Source: CAD feature listing. Evaluate the final solid. Frame: model axes, mm. Face numbers are marked on the shaded views. A direction names the side the tool comes from. Round coordinates to 2 decimals unless told otherwise and drop trailing zeros. Order: outer loops, then holes, each group sorted by start corner. A loop starts at its lowest first (then second) coordinate and runs counter-clockwise, first axis right, second up. Notation, with made-up numbers: (-35.5, -11) -> (21.5, -11) arc R4 cw to (21.5, -6) -> close; hole circle Ø1 at (80.5, -39.75). An arc over 180 degrees is marked (long way). Answer as CSV lines item,"result".
from build123d import *

# Parameters (mm, degrees)
FILLET1_R     = 10
CHAMFER1_SIZE = 2


with BuildPart() as part:
    # Sketch1 → Revolve1 (revolve)
    with BuildSketch(Plane.XY, mode=Mode.PRIVATE) as revolve1_sk:
        with BuildLine():
            Line((0, 0), (71.656242166, 0))
            ThreePointArc((71.656242166, 0), (75.656242166, 4), (79.656242166, 0))
            Line((79.656242166, 0), (148.568475549, 0))
            Line((148.568475549, 0), (148.568475549, 17))
            Line((148.568475549, 17), (79.656242166, 17))
            ThreePointArc((79.656242166, 17), (75.656242166, 13), (71.656242166, 17))
            Line((71.656242166, 17), (29.293635646, 17))
            ThreePointArc((29.293635646, 17), (20.349363736, 15.987177379), (11.858039872, 13))
            Line((11.858039872, 13), (-31.431524451, 13))
            Line((-31.431524451, 13), (-31.431524451, 0))
            Line((-31.431524451, 0), (0, 0))
        make_face()
    revolve(revolve1_sk.sketch.rotate(Axis((0, 0, 0), (1, 0, 0)), 90), axis=Axis((0, 0, 0), (1, 0, 0)))

    # Fillet1
    fillet1_edges = [part.edges().sort_by_distance(p)[0] for p in [
        (11.858039872, 0, -13),
        (-31.431524451, 0, -13),
    ]]
    fillet(fillet1_edges, radius=FILLET1_R)

    # Chamfer1
    chamfer1_edges = [part.edges().sort_by_distance(p)[0] for p in [
        (148.568475549, 0, -17),
    ]]
    chamfer(chamfer1_edges, length=CHAMFER1_SIZE)


solid = part.part
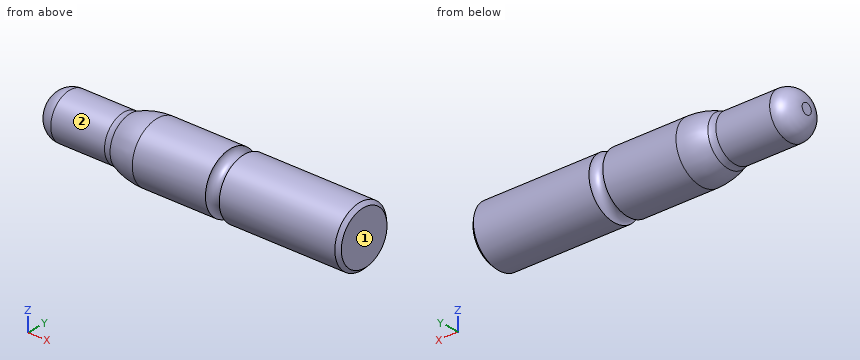
1. Reachability of the marked faces 1 and 2 from +Z, -Z, +X, -X, +Y, -Y: full face, straight path, thin tool, end or side. Return the list, or none.
Results below:
face 1,"+Z, -Z, +X, +Y, -Y"
face 2,"-X"
2. Section query A-A on x = 43. Return loops of the section in (y, z).
Results below:
outline,"circle Ø34 at (0, 0)"
3. Pin query (flat end, axial travel): pin 1 (6 mm diameter, centred on x = 116.5, z = 6.5, fed in from +Y); pin 2 (5 mm diameter, centred on x = 67, y = -6.5, fed in from +Z); pin 3 (3 mm diameter, centred on x = 110, y = -5.5, fed in from -Z); pin 4 (1.5 mm diameter, centred on y = 3.5, z = 0.5, fed in from -X). Return the tip coordinate at first contact, or that it passes through.
Results below:
pin 1,"y = 16.64"
pin 2,"z = 16.52"
pin 3,"z = -16.52"
pin 4,"x = -31.43"
4. Line query: L1, parallel to Z at x = 63, y = -0.5; L2, parallel to X at y = -13, z = 6.5; L3, parallel to X at y = 7.5, z = 12.5. Output: solid intervals per line, ascending. Write a range as [from, to].
Results below:
L1,"[-16.99, 16.99]"
L2,"[15.47, 72.51], [78.81, 148.57]"
L3,"[15.58, 72.47], [78.84, 148.57]"
